```python
from build123d import *

# Parameters (mm, degrees)
SKETCH_1_R          = 3.5
EXTRUDE_1_DEPTH     = 3
SKETCH_2_R          = 1.9
CUT_EXTRUDE_1_DEPTH = 1.5
SKETCH_3_R          = 1.25
CUT_EXTRUDE_2_DEPTH = 6.172040216
SKETCH1_R           = 1.25
SKETCH1_R_2         = 1.05
BOSS_EXTRUDE1_DEPTH = 1
SKETCH3_R           = 2
SKETCH3_R_2         = 1.25
BOSS_EXTRUDE2_DEPTH = 1


with BuildPart() as part:
    # 草图1 → 凸台-拉伸1 (new body)
    with BuildSketch(Plane.XY):
        Circle(SKETCH_1_R)
    extrude(amount=EXTRUDE_1_DEPTH)

    # 草图2 → 切除-拉伸1 (cut)
    with BuildSketch(Plane.XY.offset(3)):
        Circle(SKETCH_2_R)
    extrude(amount=-CUT_EXTRUDE_1_DEPTH, mode=Mode.SUBTRACT)

    # 草图3 → 切除-拉伸2 (cut, through all)
    with BuildSketch(Plane.XY.offset(1.5)):
        Circle(SKETCH_3_R)
    extrude(amount=-CUT_EXTRUDE_2_DEPTH, mode=Mode.SUBTRACT)



with BuildPart() as body_2:
    # Sketch1 → Boss-Extrude1 (new body)
    with BuildSketch(Plane(origin=(0, 0, 0), x_dir=(-1, 0, 0), z_dir=(0, 0, -1))):
        with Locations(Location((0, 0, 0), (0, 0, 180))):
            Circle(SKETCH1_R)
        Circle(SKETCH1_R_2, mode=Mode.SUBTRACT)
    extrude(amount=BOSS_EXTRUDE1_DEPTH)


with BuildPart() as part_1:
    add(part.part)

    add(body_2.part)  # Boss-Extrude2 merges body 2
    # Sketch3 → Boss-Extrude2 (add)
    with BuildSketch(Plane(origin=(0, 0, 0), x_dir=(-1, 0, 0), z_dir=(0, 0, -1))):
        with Locations(Location((0, 0, 0), (0, 0, 180))):
            Circle(SKETCH3_R)
        with Locations(Location((0, 0, 0), (0, 0, 180))):
            Circle(SKETCH3_R_2, mode=Mode.SUBTRACT)
    extrude(amount=BOSS_EXTRUDE2_DEPTH)


solid = part_1.part
```
Source: CAD feature listing. Evaluate the final solid. Frame: model axes, mm. A direction names the side the tool comes from. Give positions to 0.01 mm unless a question says otherwise; leave off trailing zeros. Loops run counter-clockwise (first coordinate to the right, second up) from the corner with the lowest first, then second, coordinate; pieces in that order, holes last. Notation, with made-up numbers: (41.25, 2.25) - (73.25, 2.25) arc R25 cw to (73.25, 34.25) - close; hole circle Ø4 at (31.25, 31.25). An arc over 180 degrees is marked (long way). Use CSV: the item, a comma, the result in double quotes. Start each with the question number.
1. Draft query along X for faces 1 (the cylindrical face through (-1.9, 0.08, 2.26)), 2 (the cylindrical face through (-0.434, 1.952, -0.493)), 3 (the cylindrical face through (-0.27, -1.22, 0.76)), 4 (the flat face through (2, -2, 3)). Return one class per face: +X half, -X half, draft (parallel to the pull), parting line (faces both ways), or undercut.
2. Section A-A (y = 0). Output: boundary loops of the cut face in (x, z), then the cut area to 4 significant figures.
3. Section C-C (z = -0.2). Output: boundary loops of the cut face in (x, y), then the cut area to 3 significant figures.
4. Section D-D (x = -1.5). Output: boundary loops of the cut face in (y, z), then the cut area to 3 significant figures.
5. Reachability of faces 5 (the flat face through (2, -2, 0)), 6 (the cylindrical face through (3.233, -1.341, 1.479)) from +Z, -Z, +X, -X, +Y, -Y: full face, straight path, thin tool, end or side. Return the list, or none.
6. Ray query, L1, parallel to Y at x = 0, z = 1.1; L2, parallel to Z at x = 2.75, y = 0.75; L3, parallel to Z at x = -1.5, y = -0.25. Return the intervals inside material, ascending.
7. Pin query (flat end, axial travel): pin 1 (1.2 mm diameter, centred on x = -0.5, y = 0, fed in from +Z); pin 2 (2 mm diameter, centred on y = 1.5, z = 0, fed in from -X); pin 3 (1.5 mm diameter, centred on x = -1.5, z = 0.5, fed in from -Y). Return the tip coordinate at first contact, or that it passes through.
Response:
1,face 1,"undercut"
1,face 2,"parting line"
1,face 3,"undercut"
1,face 4,"draft"
2,outline,"(-3.5, 0) - (-2, 0) - (-2, -1) - (-1.05, -1) - (-1.05, 0) - (-1.25, 0) - (-1.25, 1.5) - (-1.9, 1.5) - (-1.9, 3) - (-3.5, 3) - close; (1.05, -1) - (2, -1) - (2, 0) - (3.5, 0) - (3.5, 3) - (1.9, 3) - (1.9, 1.5) - (1.25, 1.5) - (1.25, 0) - (1.05, 0) - close"
2,area,"13.45 mm²"
3,outline,"circle Ø4 at (0, 0); hole circle Ø2.1 at (0, 0)"
3,area,"9.10 mm²"
4,outline,"(-3.16, 0) - (-1.32, 0) - (-1.32, -1) - (1.32, -1) - (1.32, 0) - (3.16, 0) - (3.16, 3) - (1.17, 3) - (1.17, 1.5) - (-1.17, 1.5) - (-1.17, 3) - (-3.16, 3) - close"
4,area,"18.1 mm²"
5,face 5,"-Z"
5,face 6,"+Z, -Z"
6,L1,"-3.5 to -1.25, 1.25 to 3.5"
6,L2,"0 to 3"
6,L3,"-1 to 1.5"
7,pin 1,"z = 0"
7,pin 2,"x = -3.46"
7,pin 3,"y = -3.42"
